from build123d import *

# Parameters (mm, degrees)
SKETCH2_W           = 30
SKETCH2_H           = 40
BOSS_EXTRUDE2_DEPTH = 25
FILLET2_R           = 1
FILLET3_R           = 1
SHELL1_START        = 2
SHELL1_OUTLINE_W    = 36
SHELL1_OUTLINE_H    = 23
SHELL1_DEPTH        = 26
FILLET4_R           = 1
SKETCH5_R           = 2
CUT_EXTRUDE10_DEPTH = 2
SKETCH7_R           = 2
BOSS_EXTRUDE3_DEPTH = 2
SKETCH4_R           = 3
CUT_EXTRUDE11_DEPTH = 2
SKETCH8_R           = 2
BOSS_EXTRUDE5_DEPTH = 2
SKETCH9_R           = 2
CUT_EXTRUDE12_DEPTH = 2
SKETCH10_R          = 2
CUT_EXTRUDE13_DEPTH = 2
SKETCH11_R          = 2
BOSS_EXTRUDE6_DEPTH = 2


# Read off the part's stored shape, not the designer's step: Shell1
with BuildPart() as part:
    # Sketch2 → Boss-Extrude2 (new body)
    with BuildSketch(Plane.XY):
        with Locations((15, 20)):
            Rectangle(SKETCH2_W, SKETCH2_H)
    extrude(amount=BOSS_EXTRUDE2_DEPTH)

    # Fillet2
    fillet2_edges = [part.edges().sort_by_distance(p)[0] for p in [
        (30, 20, 25),
        (15, 0, 25),
        (0, 20, 25),
        (15, 40, 25),
    ]]
    fillet(fillet2_edges, radius=FILLET2_R)

    # Fillet3
    # the kernel refuses this fillet: 1 mm, written as the material it takes off along each edge
    with BuildSketch(Plane(origin=(1, 39, 24), x_dir=(0, 1, 0), z_dir=(-1, 0, 0))) as fillet3_piece_1_section:
        Polygon((0, 0), (FILLET3_R, 0), (FILLET3_R, -FILLET3_R), (0, -FILLET3_R), align=None)
    fillet3_piece_1 = extrude(amount=FILLET3_R, mode=Mode.PRIVATE)
    fillet3_piece_1 = fillet3_piece_1 - Plane(origin=(1, 39, 24), x_dir=(0, -0.7071067811865475, -0.7071067811865475), z_dir=(-1, 0, 0)) * Sphere(FILLET3_R, mode=Mode.PRIVATE)
    add(fillet3_piece_1, mode=Mode.SUBTRACT)
    with BuildSketch(Plane(origin=(29, 39, 24), x_dir=(0, 1, 0), z_dir=(1, 0, 0))) as fillet3_piece_2_section:
        Polygon((0, 0), (FILLET3_R, 0), (FILLET3_R, FILLET3_R), (0, FILLET3_R), align=None)
    fillet3_piece_2 = extrude(amount=FILLET3_R, mode=Mode.PRIVATE)
    fillet3_piece_2 = fillet3_piece_2 - Plane(origin=(29, 39, 24), x_dir=(0, -0.7071067811865475, -0.7071067811865475), z_dir=(1, 0, 0)) * Sphere(FILLET3_R, mode=Mode.PRIVATE)
    add(fillet3_piece_2, mode=Mode.SUBTRACT)
    with BuildSketch(Plane(origin=(1, 1, 24), x_dir=(-1, 0, 0), z_dir=(0, -1, 0))) as fillet3_piece_3_section:
        Polygon((0, 0), (FILLET3_R, 0), (FILLET3_R, -FILLET3_R), (0, -FILLET3_R), align=None)
    fillet3_piece_3 = extrude(amount=FILLET3_R, mode=Mode.PRIVATE)
    fillet3_piece_3 = fillet3_piece_3 - Plane(origin=(1, 1, 24), x_dir=(0.7071067811865475, 0, -0.7071067811865475), z_dir=(0, -1, 0)) * Sphere(FILLET3_R, mode=Mode.PRIVATE)
    add(fillet3_piece_3, mode=Mode.SUBTRACT)
    with BuildSketch(Plane(origin=(29, 1, 24), x_dir=(1, 0, 0), z_dir=(0, -1, 0))) as fillet3_piece_4_section:
        Polygon((0, 0), (FILLET3_R, 0), (FILLET3_R, FILLET3_R), (0, FILLET3_R), align=None)
    fillet3_piece_4 = extrude(amount=FILLET3_R, mode=Mode.PRIVATE)
    fillet3_piece_4 = fillet3_piece_4 - Plane(origin=(29, 1, 24), x_dir=(-0.7071067811865475, 0, -0.7071067811865475), z_dir=(0, -1, 0)) * Sphere(FILLET3_R, mode=Mode.PRIVATE)
    add(fillet3_piece_4, mode=Mode.SUBTRACT)
    with BuildSketch(Plane(origin=(30, 0, -2.5), x_dir=(-1, 0, 0), z_dir=(0, 0, 1)), Plane(origin=(30, 40, -2.5), x_dir=(0, -1, 0), z_dir=(0, 0, 1))) as fillet3_piece_5:
        with BuildLine():
            CenterArc((FILLET3_R, -FILLET3_R), FILLET3_R, 90, 90)
            Line((0, -FILLET3_R), (0, 0))
            Line((0, 0), (FILLET3_R, 0))
        make_face()
    extrude(amount=26.5, mode=Mode.SUBTRACT)
    with BuildSketch(Plane(origin=(0, 0, -2.5), x_dir=(1, 0, 0), z_dir=(0, 0, 1)), Plane(origin=(0, 40, -2.5), x_dir=(0, -1, 0), z_dir=(0, 0, 1))) as fillet3_piece_6:
        with BuildLine():
            CenterArc((FILLET3_R, FILLET3_R), FILLET3_R, 180, 90)
            Line((0, FILLET3_R), (0, 0))
            Line((0, 0), (FILLET3_R, 0))
        make_face()
    extrude(amount=26.5, mode=Mode.SUBTRACT)

    # Shell1 outline → Shell1 (cut)
    with BuildSketch(Plane.YZ.offset(SHELL1_START)):
        with Locations((20, 11.5)):
            Rectangle(SHELL1_OUTLINE_W, SHELL1_OUTLINE_H)
    extrude(amount=SHELL1_DEPTH, mode=Mode.SUBTRACT)

    # Fillet4
    fillet4_edges = [part.edges().sort_by_distance(p)[0] for p in [
        (28, 20, 23),
        (2, 20, 23),
        (15, 2, 23),
        (15, 38, 23),
    ]]
    fillet(fillet4_edges, radius=FILLET4_R)

    # Sketch5 → Cut-Extrude10 (cut)
    with BuildSketch(Plane.XZ):
        with Locations(Location((20, 17.5, 0), (0, 0, 270))):
            Circle(SKETCH5_R)
        with Locations(Location((10, 7.5, 0), (0, 0, 270))):
            Circle(SKETCH5_R)
    extrude(amount=-CUT_EXTRUDE10_DEPTH, mode=Mode.SUBTRACT)

    # Sketch7 → Boss-Extrude3 (add)
    with BuildSketch(Plane(origin=(0, 0, 0), x_dir=(-1, 0, 0), z_dir=(0, -1, 0))):
        with Locations(Location((-10, -17.5, 0), (0, 0, 270))):
            Circle(SKETCH7_R)
        with Locations(Location((-20, -7.5, 0), (0, 0, 270))):
            Circle(SKETCH7_R)
    extrude(amount=BOSS_EXTRUDE3_DEPTH)

    # Sketch4 → Cut-Extrude11 (cut)
    with BuildSketch(Plane.XY.offset(25)):
        with Locations((15, 25)):
            Circle(SKETCH4_R)
    extrude(amount=-CUT_EXTRUDE11_DEPTH, mode=Mode.SUBTRACT)

    # Sketch8 → Boss-Extrude5 (add)
    with BuildSketch(Plane(origin=(30, 0, 0), x_dir=(0, 0, -1), z_dir=(1, 0, 0))):
        with Locations(Location((-7.5, 25, 0), (0, 0, 270))):
            Circle(SKETCH8_R)
        with Locations(Location((-17.5, 15, 0), (0, 0, 270))):
            Circle(SKETCH8_R)
    extrude(amount=BOSS_EXTRUDE5_DEPTH)

    # Sketch9 → Cut-Extrude12 (cut)
    with BuildSketch(Plane(origin=(30, 0, 0), x_dir=(0, 0, -1), z_dir=(1, 0, 0))):
        with Locations(Location((-7.5, 15, 0), (0, 0, 90))):
            Circle(SKETCH9_R)
        with Locations(Location((-17.5, 25, 0), (0, 0, 90))):
            Circle(SKETCH9_R)
    extrude(amount=-CUT_EXTRUDE12_DEPTH, mode=Mode.SUBTRACT)

    # Sketch10 → Cut-Extrude13 (cut)
    with BuildSketch(Plane.ZY):
        with Locations(Location((7.5, 25, 0), (0, 0, 270))):
            Circle(SKETCH10_R)
        with Locations(Location((16.5, 15, 0), (0, 0, 270))):
            Circle(SKETCH10_R)
    extrude(amount=-CUT_EXTRUDE13_DEPTH, mode=Mode.SUBTRACT)

    # Sketch11 → Boss-Extrude6 (add)
    with BuildSketch(Plane.ZY):
        with Locations(Location((16.5, 25, 0), (0, 0, 270))):
            Circle(SKETCH11_R)
        with Locations(Location((7.5, 15, 0), (0, 0, 90))):
            Circle(SKETCH11_R)
    extrude(amount=BOSS_EXTRUDE6_DEPTH)


solid = part.part
For this review, take the finished solid that the model builds, in its own axes (mm). A direction names the side the tool comes from. Round coordinates to 2 decimals unless told otherwise and drop trailing zeros. Loops run counter-clockwise (first coordinate to the right, second up) from the corner with the lowest first, then second, coordinate; pieces in that order, holes last. Notation, with made-up numbers: (49, -13.5) - (76, -13.5) arc R22 ccw to (76, 11.5) - close; hole circle Ø2 at (2, 67.5). An arc over 180 degrees is marked (long way). Use one line per item in the form item = value.
Item 1: Tool access review of faces 4 (the flat face through (2, 20, 11)), 5 (the cylindrical face through (8.648, -0.986, 16.026)), 6 (the cylindrical face through (29.014, 24.74, 19.483)): name each direction out of +Z, -Z, +X, -X, +Y, -Y from which nothing blocks a thin tool from reaching the whole face with its end or side.
Answers:
face_4 = -Z
face_5 = -Y
face_6 = +X
Item 2: Consider section B-B on x = 20. Write out the cut boundary in (y, z), then the cut area to 3 significant figures.
Answers:
outline = (-2, 5.5) - (0, 5.5) - (0, 0) - (2, 0) - (2, 15.5) - (0, 15.5) - (0, 9.5) - (-2, 9.5) - close; (0, 19.5) - (2, 19.5) - (2, 22) arc R1 cw to (3, 23) - (37, 23) arc R1 cw to (38, 22) - (38, 0) - (40, 0) - (40, 24) arc R1 ccw to (39, 25) - (1, 25) arc R1 ccw to (0, 24) - close
area = 172 mm^2
Item 3: Consider section C-C on y = 15. Write out the cut boundary in (x, z).
Answers:
outline = (-2, 5.5) - (0, 5.5) - (0, 0) - (2, 0) - (2, 14.5) - (0, 14.5) - (0, 9.5) - (-2, 9.5) - close; (0, 18.5) - (2, 18.5) - (2, 22) arc R1 cw to (3, 23) - (27, 23) arc R1 cw to (28, 22) - (28, 9.5) - (30, 9.5) - (30, 15.5) - (32, 15.5) - (32, 19.5) - (30, 19.5) - (30, 24) arc R1 ccw to (29, 25) - (1, 25) arc R1 ccw to (0, 24) - close; (28, 0) - (30, 0) - (30, 5.5) - (28, 5.5) - close
Item 4: Consider section A-A on y = 25. State how many separate pieces and enclosed holes the cut face has, then the cut area to 3 significant figures.
Answers:
separate_pieces = 4
enclosed_holes = 0
area = 140 mm^2
Item 5: For line 1 (X direction, y = 22.5, z = 4.75); line 2 (Y direction, x = 13.5, z = 7); line 3 (X direction, y = 1.2, z = 17.5), list the stretches that pass through material, from the lowest coordinate up.
Answers:
line_1 = 0 to 2, 28 to 30
line_2 = 0 to 2, 38 to 40
line_3 = 0 to 18, 22 to 30
Item 6: Consider section D-D on z = 23.5. Write out the cut boundary in (x, y).
Answers:
outline = (0, 1) arc R1 ccw to (1, 0) - (29, 0) arc R1 ccw to (30, 1) - (30, 39) arc R1 ccw to (29, 40) - (1, 40) arc R1 ccw to (0, 39) - close; hole circle Ø6 at (15, 25)
Item 7: Clearance check with flat-ended pins moving along their axes: P1, Ø6.5, axis at y = 17.5, z = 6, coming from the +X side; P2, Ø12, axis at x = 15, z = 6.5, coming from the -Y side; P3, Ø3.5, axis at y = 25, z = 7.5, coming from the -X side; P4, Ø2, axis at y = 21.5, z = 5.5, coming from the -X side. State where each tip first meets the part, or that it passes through.
Answers:
P1 = 30
P2 = -2
P3 = 28
P4 = 0
Item 8: Mouldability with a two-part tool opening along Z and no side actions: class faces 1 (the cylindrical face through (27.715, 20.252, 22.699)), 2 (the flat face through (20, -2, 7)), 3 (the cylindrical face through (0.986, 15.26, 18.483)) as +Z half, -Z half, draft (parallel to the pull), parting line (faces both ways), or undercut.
Answers:
face_1 = -Z half
face_2 = draft
face_3 = undercut
